```python
from build123d import *

# Parameters (mm, degrees)
CYLINDER003_R           = 1.3
CYLINDER003_DEPTH       = 10
CYLINDER001_R           = 1.5
CYLINDER001_DEPTH       = 3
CYLINDER001_PITCH_ANGLE = 90
CYLINDER_R              = 1.5
CYLINDER_DEPTH          = 3
CYLINDER_PITCH_ANGLE    = 90
CYLINDER002_R           = 3
CYLINDER002_DEPTH       = 8
BOX001_W                = 3
BOX001_H                = 10
BOX001_DEPTH            = 15
BOX002_W                = 3
BOX002_H                = 10
BOX002_DEPTH            = 15
BOX_W                   = 21
BOX_H                   = 10
BOX_DEPTH               = 3


with BuildPart() as cylinder001:
    # Cylinder003 → Cylinder003 (new body)
    with BuildSketch(Plane(origin=(10.5, 5, -7), x_dir=(1, 0, 0), z_dir=(0, 0, 1))):
        Circle(CYLINDER003_R)
    extrude(amount=CYLINDER003_DEPTH)


with BuildPart() as hole002:
    # Cylinder001 → Cylinder001 (new body)
    with BuildSketch(Plane.XY):
        Circle(CYLINDER001_R)
    extrude(amount=CYLINDER001_DEPTH)


with BuildPart() as hole002_1:
    # Cylinder001 pitch: moved
    add(hole002.part.rotate(Axis((0, 0, 0), (0, 1, 0)), CYLINDER001_PITCH_ANGLE))


with BuildPart() as hole002_2:
    # Cylinder001 placement: moved
    add(hole002_1.part.moved(Location((18, 5, 13))))


with BuildPart() as hole1:
    # Cylinder → Cylinder (new body)
    with BuildSketch(Plane.XY):
        Circle(CYLINDER_R)
    extrude(amount=CYLINDER_DEPTH)


with BuildPart() as hole1_1:
    # Cylinder pitch: moved
    add(hole1.part.rotate(Axis((0, 0, 0), (0, 1, 0)), CYLINDER_PITCH_ANGLE))


with BuildPart() as hole1_2:
    # Cylinder placement: moved
    add(hole1_1.part.moved(Location((0, 5, 13))))


with BuildPart() as cylinder:
    # Cylinder002 → Cylinder002 (new body)
    with BuildSketch(Plane(origin=(10.5, 5, -7), x_dir=(1, 0, 0), z_dir=(0, 0, 1))):
        Circle(CYLINDER002_R)
    extrude(amount=CYLINDER002_DEPTH)


with BuildPart() as cube001:
    # Box001 → Box001 (new body)
    with BuildSketch(Plane.XY):
        with Locations((1.5, 5)):
            Rectangle(BOX001_W, BOX001_H)
    extrude(amount=BOX001_DEPTH)


with BuildPart() as cube002:
    # Box002 → Box002 (new body)
    with BuildSketch(Plane(origin=(18, 0, 0), x_dir=(1, 0, 0), z_dir=(0, 0, 1))):
        with Locations((1.5, 5)):
            Rectangle(BOX002_W, BOX002_H)
    extrude(amount=BOX002_DEPTH)


with BuildPart() as cut002:
    # Box → Box (new body)
    with BuildSketch(Plane.XY):
        with Locations((10.5, 5)):
            Rectangle(BOX_W, BOX_H)
    extrude(amount=BOX_DEPTH)

    # Fusion: union Cube001, Cube002
    add(cube001.part)
    add(cube002.part)

    # Fusion001: union Cylinder
    add(cylinder.part)

    # Cut: cut Hole1
    add(hole1_2.part, mode=Mode.SUBTRACT)

    # Cut001: cut Hole002
    add(hole002_2.part, mode=Mode.SUBTRACT)

    # Cut002: cut Cylinder001
    add(cylinder001.part, mode=Mode.SUBTRACT)


solid = cut002.part
```
The model under review builds one solid part; all positions refer to its coordinate system, in mm. A direction names the side the tool comes from. Round coordinates to 2 decimals unless told otherwise and drop trailing zeros. Loops run counter-clockwise (first coordinate to the right, second up) from the corner with the lowest first, then second, coordinate; pieces in that order, holes last.
Item 1: Take a section at A-A (x = 10.5). Write out the cut boundary in (y, z), then the cut area to 3 significant figures.
Determined:
outline: (0, 0) - (2, 0) - (2, -7) - (3.7, -7) - (3.7, 3) - (0, 3) - close; (6.3, -7) - (8, -7) - (8, 0) - (10, 0) - (10, 3) - (6.3, 3) - close
area: 46.0 mm2
Item 2: Mouldability with a two-part tool opening along Z and no side actions: class faces 1 (the face through (19.48, 5.07, 14.5)), 2 (the face through (8, 7, 0)), 3 (the face through (19, 5, 15)) as released by +Z, released by -Z, zero draft, split by the parting line, or undercut.
Determined:
face 1: undercut
face 2: released by -Z
face 3: released by +Z
Item 3: For line 1 (Y direction, x = 1.1, z = 13); line 2 (Y direction, x = 10.5, z = -4.75); line 3 (X direction, y = 8.5, z = 10.25), list the stretches that pass through material, from the lowest coordinate up.
Determined:
line 1: y = 0 to 3.5, 6.5 to 10
line 2: y = 2 to 3.7, 6.3 to 8
line 3: x = 0 to 3, 18 to 21
Item 4: For faces 4 (the face through (0, 5, 7)), 5 (the face through (9.85, 2.07, -3.55)), 6 (the face through (12, 5, 3)), list the 3-axis set-ups (+Z, -Z, +X, -X, +Y, -Y) from which the entire face can be reached by the end or side of a thin tool; tool diameter is ignored.
Determined:
face 4: +Z, -Z, -X, +Y, -Y
face 5: -Z
face 6: +Z, +Y, -Y
Item 5: Take a section at B-B (z = 13). Write out the cut boundary in (x, y), then the cut area to 3 significant figures.
Determined:
outline: (0, 0) - (3, 0) - (3, 3.5) - (0, 3.5) - close; (0, 6.5) - (3, 6.5) - (3, 10) - (0, 10) - close; (18, 0) - (21, 0) - (21, 3.5) - (18, 3.5) - close; (18, 6.5) - (21, 6.5) - (21, 10) - (18, 10) - close
area: 42.0 mm2
Item 6: Clearance check with flat-ended pins moving along their axes: pin 1 Ø1 at (x, y) = (12, 7.5) entering from +Z; pin 2 Ø2 at (x, y) = (14.5, 3) entering from -Z; pin 3 Ø6 at (y, z) = (4.5, -4.5) entering from +X. State where each tip first meets the part, or that it passes through.
Determined:
pin 1: stops at z = 3
pin 2: stops at z = 0
pin 3: stops at x = 13.5
Item 7: Take a section at C-C (z = 3.5). Write out the cut boundary in (x, y), then the cut area to 3 significant figures.
Determined:
outline: (0, 0) - (3, 0) - (3, 10) - (0, 10) - close; (18, 0) - (21, 0) - (21, 10) - (18, 10) - close
area: 60.0 mm2
Item 8: Take a section at D-D (y = 5). Write out the cut boundary in (x, z), then the cut area to 3 significant figures.
Determined:
outline: (0, 0) - (7.5, 0) - (7.5, -7) - (9.2, -7) - (9.2, 3) - (3, 3) - (3, 11.5) - (0, 11.5) - close; (0, 14.5) - (3, 14.5) - (3, 15) - (0, 15) - close; (11.8, -7) - (13.5, -7) - (13.5, 0) - (21, 0) - (21, 11.5) - (18, 11.5) - (18, 3) - (11.8, 3) - close; (18, 14.5) - (21, 14.5) - (21, 15) - (18, 15) - close
area: 133 mm2
